from build123d import *

# Parameters (mm, degrees)
F0_W     = 24.9
F0_H     = 10
F1_DEPTH = 10
F4_DEPTH = 24.901
F5_DEPTH = 10.001


with BuildPart() as f1:
    # F0 (on Front) → F1 (new body)
    with BuildSketch(Plane.XZ):
        Rectangle(F0_W, F0_H)
    extrude(amount=F1_DEPTH)

    # F3 (on face) → F4 (cut, through all)
    with BuildSketch(Plane(origin=(-12.45, 0, 0), x_dir=(0, -1, 0), z_dir=(-1, 0, 0))):
        with BuildLine():
            ThreePointArc((0, 0), (1.4644660941, 3.5355339059), (5, 5))
            Line((5, 5), (0, 5))
            Line((0, 5), (0, 0))
        make_face()
        with BuildLine():
            ThreePointArc((5, 5), (8.5355339059, 3.5355339059), (10, 0))
            Line((10, 0), (10, 5))
            Line((10, 5), (5, 5))
        make_face()
        with BuildLine():
            Line((0, -5), (5, -5))
            ThreePointArc((5, -5), (1.4644660941, -3.5355339059), (0, 0))
            Line((0, 0), (0, -5))
        make_face()
        with BuildLine():
            Line((10, -5), (10, 0))
            ThreePointArc((10, 0), (8.5355339059, -3.5355339059), (5, -5))
            Line((5, -5), (10, -5))
        make_face()
    extrude(amount=-F4_DEPTH, mode=Mode.SUBTRACT)

    # F2 (on face) → F5 (cut, through all)
    with BuildSketch(Plane.XZ.offset(10)):
        with BuildLine():
            ThreePointArc((-12.45, 0), (-12.1851488571, 2.5543389223), (-11.4018638827, 5))
            Line((-11.4018638827, 5), (-12.45, 5))
            Line((-12.45, 5), (-12.45, 0))
        make_face()
        with BuildLine():
            Line((-12.45, -5), (-11.4018638827, -5))
            ThreePointArc((-11.4018638827, -5), (-12.1851488571, -2.5543389223), (-12.45, 0))
            Line((-12.45, 0), (-12.45, -5))
        make_face()
        with BuildLine():
            ThreePointArc((11.4018638827, 5), (12.1851488571, 2.5543389223), (12.45, 0))
            Line((12.45, 0), (12.45, 5))
            Line((12.45, 5), (11.4018638827, 5))
        make_face()
        with BuildLine():
            Line((12.45, -5), (12.45, 0))
            ThreePointArc((12.45, 0), (12.1851488571, -2.5543389223), (11.4018638827, -5))
            Line((11.4018638827, -5), (12.45, -5))
        make_face()
    extrude(amount=-F5_DEPTH, mode=Mode.SUBTRACT)


solid = f1.part
Geometry check sheet. Reference: the model listing, model coordinates, mm. Give positions to 0.01 mm unless a question says otherwise; leave off trailing zeros. Order: outer loops, then holes, each group sorted by start corner. A loop starts at its lowest first (then second) coordinate and runs counter-clockwise, first axis right, second up.
1) Cross-section at D-D (y = -9). Record the boundary of the cut face in (x, z).
Results are:
outline: (-12.08, -3) - (12.08, -3) arc R12.45 ccw to (12.08, 3) - (-12.08, 3) arc R12.45 ccw to start
2) Cross-section at B-B (x = 5.75). Record the boundary of the cut face in (y, z), then the cut area to 3 significant figures.
Results are:
outline: circle Ø10 at (-5, 0)
area: 78.5 mm2
3) Cross-section at C-C (z = -1.75). Record the boundary of the cut face in (x, y).
Results are:
outline: (-12.33, -9.68) - (12.33, -9.68) - (12.33, -0.32) - (-12.33, -0.32) - close
4) Material ranges on probe 1 along X at (y, z) = (-4, -0.25); probe 2 along Y at (x, z) = (-9.5, -0.25); probe 3 along Y at (x, z) = (-1, 0.75), recorded low to high.
Results are:
probe 1: x = -12.45 to 12.45
probe 2: y = -9.99 to -0.01
probe 3: y = -9.94 to -0.06
5) Cross-section at A-A (y = -0.75). Record the boundary of the cut face in (x, z), then the cut area to 3 significant figures.
Results are:
outline: (-12.17, -2.63) - (12.17, -2.63) arc R12.45 ccw to (12.17, 2.63) - (-12.17, 2.63) arc R12.45 ccw to start
area: 130 mm2
6) Gauge pin test, flat ends, axial feed: pin 1 (1.5 mm diameter, centred on x = 2, y = -6, fed in from +Z); pin 2 (1.5 mm diameter, centred on y = -3, z = -1, fed in from -X); pin 3 (2 mm diameter, centred on x = 1, y = -3, fed in from +Z). Record the tip position at first contact, or that the pin passes through.
Results are:
pin 1: stops at z = 4.99
pin 2: stops at x = -12.45
pin 3: stops at z = 4.9
